Model file for the job. Use its own axes, mm. A direction names the side the tool comes from. Coordinates: 2 decimals unless noted, no trailing zeros. Write each loop counter-clockwise with the first axis right and the second up, starting at its lowest first coordinate (ties: lowest second). Pieces come first, ordered by that corner, then holes. Notation, with made-up numbers: (70, 88.25) - (128, 88.25) arc R36 ccw to (128, 122.25) - close; hole circle Ø2 at (83.25, 26). An arc over 180 degrees is marked (long way). Put each result on its own line as item: value. Start each with the question number.
1. Drop flat-ended pins along their axis: P1, Ø2, axis at y = 7.5, z = 0.5, coming from the +X side; P2, Ø14, axis at x = 10, y = 8.5, coming from the +Z side; P3, Ø10, axis at x = -7.5, y = -5.5, coming from the -Z side; P4, Ø1, axis at x = -6.5, z = 2, coming from the -Y side. Give the stop position or say it passes through.
2. Saw through at D-D, the plane x = 6.5. Write the cut outline in (y, z).
3. Saw through at B-B, the plane x = 0. Write the cut outline in (y, z).
4. Saw through at C-C, the plane z = 2.95. Write the cut outline in (x, y), plus the area to 3 significant figures.
5. Which spindle directions (+Z, -Z, +X, -X, +Y, -Y) get a long thin tool onto all of the face, cutting with end or side? Do faces 4 (the face through (-7, 0, 3.6)), 5 (the face through (5, 0, 2)). Say none if no direction does.
6. Pull direction X, two halves, no side cores. Call faces 1 (the face through (-2.994, -22.804, 0.296)), 2 (the face through (0, -5, 0)), 3 (the face through (-8, 0, 2)): released by +X, released by -X, zero draft, split by the parting line, or undercut.
7. Drill centre lines: L1, parallel to Y at x = 0, z = 0.15; L2, parallel to Z at x = -11.5, y = -13; L3, parallel to X at y = -12.5, z = 0.2. Where is each one in solid material? Low to high. Write a range as from..to.
8. Saw through at A-A, the plane y = 0. Write the cut outline in (x, z).
Autodesk Inventor part; units mm, degrees
ref_plane "YZ Plane" through (0, 0, 0) normal (1, 0, 0) x (0, 1, 0)
ref_plane "XZ Plane" through (0, 0, 0) normal (0, 1, 0) x (-1, 0, 0)
ref_plane "XY Plane" through (0, 0, 0) normal (0, 0, 1) x (1, 0, 0)
sketch "スケッチ1" plane through (0, 0, 0) normal (0, 0, 1) x (1, 0, 0)
  circle A0 centre (0, 0) radius 23
  circle A1 centre (0, 0) radius 4
  dimension "d0" = 46
  dimension "d1" = 8
extrude "押し出し1" add sketch "スケッチ1" along normal blind 0.6
sketch "スケッチ2" plane through (0, 0, 0.6) normal (0, 0, 1) x (1, 0, 0)
  circle A0 centre (0, 0) radius 6.5 construction
  circle A1 centre (-6.5, 0) radius 1.5
  circle A2 centre (6.5, 0) radius 1.5
  dimension "d4" = 13
  dimension "d5" = 3
extrude "押し出し2" add sketch "スケッチ2" along normal blind 3
properties part number "SlitDiscSupport2"
Final values:
1. P1: stops at x = 22.06
1. P2: stops at z = 0.6
1. P3: stops at z = 0
1. P4: stops at y = -1.5
2. outline: (-22.06, 0) - (22.06, 0) - (22.06, 0.6) - (1.5, 0.6) - (1.5, 3.6) - (-1.5, 3.6) - (-1.5, 0.6) - (-22.06, 0.6) - close
3. outline: (-23, 0) - (-4, 0) - (-4, 0.6) - (-23, 0.6) - close; (4, 0) - (23, 0) - (23, 0.6) - (4, 0.6) - close
4. outline: circle Ø3 at (-6.5, 0); circle Ø3 at (6.5, 0)
4. area: 14.1 mm²
5. face 4: +Z, +X, -X, +Y, -Y
5. face 5: +Z
6. face 1: split by the parting line
6. face 2: zero draft
6. face 3: undercut
7. L1: y = -23..-4, 4..23
7. L2: z = 0..0.6
7. L3: x = -19.31..19.31
8. outline: (-23, 0) - (-4, 0) - (-4, 0.6) - (-5, 0.6) - (-5, 3.6) - (-8, 3.6) - (-8, 0.6) - (-23, 0.6) - close; (4, 0) - (23, 0) - (23, 0.6) - (8, 0.6) - (8, 3.6) - (5, 3.6) - (5, 0.6) - (4, 0.6) - close
